```python
from build123d import *

# Parameters (mm, degrees)
PAD013_DEPTH    = 2.25
SKETCH022_R     = 0.65
PAD014_DEPTH    = 1.6
CHAMFER003_SIZE = 0.2


with BuildPart() as part:
    # Sketch020 → Pad013 (new body, symmetric)
    with BuildSketch(Plane.YZ):
        with BuildLine():
            Line((0, 0), (0, 5.3))
            Line((0, 5.3), (-1.25, 5.3))
            Line((-1.25, 5.3), (-3.159701, 3.065466))
            ThreePointArc((-4.3, 2.54), (-3.672227, 2.677686), (-3.159701, 3.065466))
            Line((-4.3, 2.54), (-6.4, 2.54))
            Line((-6.4, 2.54), (-6.4, 0))
            Line((-6.4, 0), (-4.3, 0))
            Line((-4.3, 0), (-4.3, 1.5))
            Line((-4.3, 1.5), (-0.7, 1.5))
            Line((-0.7, 1.5), (-0.7, 0))
            Line((-0.7, 0), (0, 0))
        make_face()
    extrude(amount=PAD013_DEPTH, both=True)

    # Sketch021 → Revolution (revolve)
    with BuildSketch(Plane.YZ):
        with BuildLine():
            Line((0, 3.8), (2.54, 3.8))
            ThreePointArc((2.54, 3.8), (2.10066, 4.86066), (1.04, 5.3))
            Line((1.04, 5.3), (0, 5.3))
            Line((0, 5.3), (0, 3.8))
        make_face()
    revolve(axis=Axis((0, 2.54, 3.8), (0, 1, 0)))

    # Sketch022 → Pad014 (join)
    with BuildSketch(Plane.XY):
        with Locations((-1.27, -5.2)):
            Circle(SKETCH022_R)
    pad014 = extrude(amount=-PAD014_DEPTH)

    # Mirrored003: Pad014 across Sketch022 V_Axis
    add(pad014.mirror(Plane(origin=(0, 0, 0), x_dir=(0, 0, 1), z_dir=(1, 0, 0))))

    # Chamfer003
    chamfer003_edges = [part.edges().sort_by_distance(p)[0] for p in [
        (1.92, -5.2, -1.6),
        (-1.92, -5.2, -1.6),
    ]]
    chamfer(chamfer003_edges, length=CHAMFER003_SIZE)


solid = part.part
```
Check sheet for the modelled part. Datum: model origin and axes. Units: mm. A direction names the side the tool comes from. Coordinates: 2 decimals unless noted, no trailing zeros. Write each loop counter-clockwise with the first axis right and the second up, starting at its lowest first coordinate (ties: lowest second). Pieces come first, ordered by that corner, then holes. Notation, with made-up numbers: M 58.5,33 L 101.5,33 A32 cw 101.5,62 Z; hole C -26,-17.75 d4. An arc over 180 degrees is marked long. Use one line per item in the form item = value.
Item 1: Sectioned sample at B-B, the plane y = -5.2. Record the cut outline in (x, z).
Answer below:
outline = M -2.25,0 L -1.92,0 L -1.92,-1.4 L -1.72,-1.6 L -0.82,-1.6 L -0.62,-1.4 L -0.62,0 L 0.62,0 L 0.62,-1.4 L 0.82,-1.6 L 1.72,-1.6 L 1.92,-1.4 L 1.92,0 L 2.25,0 L 2.25,2.54 L -2.25,2.54 Z
Item 2: Sectioned sample at A-A, the plane z = 0.25. Record the cut outline in (x, y).
Answer below:
outline = M -2.25,-6.4 L 2.25,-6.4 L 2.25,-4.3 L -2.25,-4.3 Z; M -2.25,-0.7 L 2.25,-0.7 L 2.25,0 L -2.25,0 Z
Item 3: Gauge pin test, flat ends, axial feed: pin 1 Ø0.6 at (x, y) = (-1, -5) entering from +Z; pin 2 Ø1.8 at (x, y) = (0.5, -2.5) entering from -Z; pin 3 Ø0.8 at (x, z) = (0.5, 1) entering from +Y. Record the tip position at first contact, or that the pin passes through.
Answer below:
pin_1 = 2.54
pin_2 = 1.5
pin_3 = 0
Item 4: Sectioned sample at C-C, the plane z = -0.5. Record the cut outline in (x, y), and give its area (3 significant figures).
Answer below:
outline = C -1.27,-5.2 d1.3; C 1.27,-5.2 d1.3
area = 2.65 mm^2
Item 5: Sectioned sample at D-D, the plane z = 2. Record the cut outline in (x, y).
Answer below:
outline = M -2.25,-6.4 L 2.25,-6.4 L 2.25,0 L -2.25,0 Z
Item 6: Material ranges on L1, parallel to X at y = -5.25, z = -0.25; L2, parallel to Y at x = 1.6, z = 0.5; L3, parallel to Y at x = -1.9, z = 2.5, recorded low to high. Write a range as from..to.
Answer below:
L1 = -1.92..-0.62, 0.62..1.92
L2 = -6.4..-4.3, -0.7..0
L3 = -6.4..0
Item 7: Set-up check for faces 1 (the face through (0, -5, 2.54)), 2 (the face through (-1.411, -5.835, -0.69)), 3 (the face through (0, -3, 1.5)): record each of +Z, -Z, +X, -X, +Y, -Y from which the full face is reachable in a straight line by a thin tool's end or side.
Answer below:
face_1 = +Z, +X, -X, -Y
face_2 = -Z
face_3 = -Z, +X, -X
